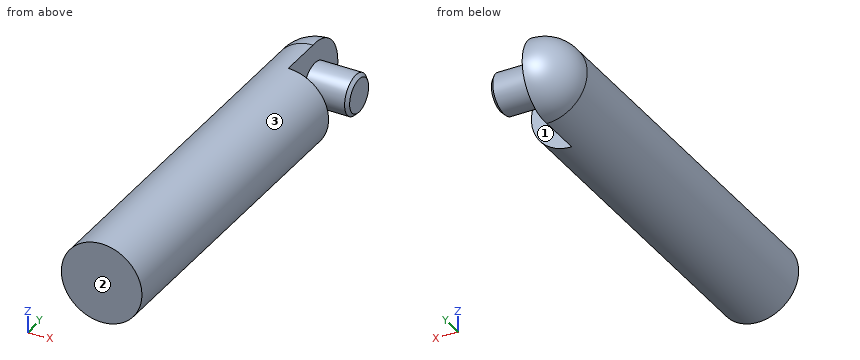
```python
from build123d import *

# Parameters (mm, degrees)
SKETCH1_R               = 19.05
BOSS_EXTRUDE1_DEPTH     = 177.8
DOME1_FACE_RADIUS       = 19.05
DOME1_HEIGHT            = 20.828
CUT_EXTRUDE1_DEPTH      = 201.461172648
CUT_EXTRUDE1_DEPTH_BACK = 201.461172648
SKETCH2_W               = 31.75
SKETCH2_H               = 41.656
SKETCH3_R               = 9.525
BOSS_EXTRUDE2_DEPTH     = 20.828
CHAMFER1_SIZE           = 1.524


with BuildPart() as part:
    # Sketch1 → Boss-Extrude1 (new body)
    with BuildSketch(Plane(origin=(0, 0, 0), x_dir=(1, 0, 0), z_dir=(0, 1, 0))):
        with Locations(Location((0, 0, 0), (0, 0, 270))):
            Circle(SKETCH1_R)
    extrude(amount=BOSS_EXTRUDE1_DEPTH)

    # Dome1: a dome of height H over a round flat face of radius A is a cap of a sphere of radius (A * A + H * H) / (2 * H)
    dome1_r = (DOME1_FACE_RADIUS * DOME1_FACE_RADIUS + DOME1_HEIGHT * DOME1_HEIGHT) / (2 * DOME1_HEIGHT)
    dome1_base = Plane((0, 177.8, 0), z_dir=(0, 1, 0))
    with Locations(dome1_base.offset(DOME1_HEIGHT - dome1_r)):
        dome1_ball = Sphere(dome1_r, mode=Mode.PRIVATE)
    add(split(dome1_ball, bisect_by=dome1_base, keep=Keep.TOP, mode=Mode.PRIVATE))

    # Sketch2 → Cut-Extrude1 (cut, two sides: drawn at the far end of the back side and taken through both)
    with BuildSketch(Plane.XY.offset(-CUT_EXTRUDE1_DEPTH_BACK)):
        with Locations((15.875, 177.8)):
            Rectangle(SKETCH2_W, SKETCH2_H)
    extrude(amount=CUT_EXTRUDE1_DEPTH + CUT_EXTRUDE1_DEPTH_BACK, mode=Mode.SUBTRACT)

    # Sketch3 → Boss-Extrude2 (add)
    with BuildSketch(Plane(origin=(0, 0, 0), x_dir=(0, 0, -1), z_dir=(1, 0, 0))):
        with Locations(Location((0, 179.502109756, 0), (0, 0, 270))):
            Circle(SKETCH3_R)
    extrude(amount=BOSS_EXTRUDE2_DEPTH)

    # Chamfer1
    chamfer1_edges = [part.edges().sort_by_distance(p)[0] for p in [
        (20.828, 189.027109756, 0),
    ]]
    chamfer(chamfer1_edges, length=CHAMFER1_SIZE)


solid = part.part
```
Design review of the part built by this model. Coordinates are the model's own, in mm. Face numbers are marked on the shaded views. Coordinates: 2 decimals unless noted, no trailing zeros. Order: outer loops, then holes, each group sorted by start corner. A loop starts at its lowest first (then second) coordinate and runs counter-clockwise, first axis right, second up.
1) Wall thickness on line 1 along Y through (x, z) = (6.5, -0.5); line 2 along Y through (x, z) = (17, -8.5); line 3 along Z through (x, y) = (-16.5, 135): over which ranges is each line inside the solid? List them lowest first.
2) Take a section at D-D, the plane x = 16.5. Give the boundary of the cut face in (y, z) (3 decimals).
3) Mouldability with a two-part tool opening along Y and no side actions: class the marked faces 1, 2 and 3 as +Y half, -Y half, draft (parallel to the pull), parting line (faces both ways), or undercut.
4) Take a section at C-C, the plane y = 126. Give the boundary of the cut face in (x, z).
5) Take a section at A-A, the plane z = 0. Give the boundary of the cut face in (x, y).
6) Clearance check with flat-ended pins moving along their axes: pin 1 (2 mm diameter, centred on x = -2.5, y = 144.5, fed in from -Z); pin 2 (8 mm diameter, centred on y = 65, z = 5, fed in from -X); pin 3 (3 mm diameter, centred on x = 0, z = 13.5, fed in from -Y); pin 4 (2 mm diameter, centred on x = 5.5, y = 20.5, fed in from +Z). State where each tip first meets the part, or that it passes through.
7) Take a section at B-B, the plane x = 8. Give the boundary of the cut face in (y, z) (3 decimals).
Returned:
1. line 1: y = 0 to 156.97, 169.99 to 189.01
1. line 2: y = 0 to 156.97, 175.2 to 183.8
1. line 3: z = -9.52 to 9.52
2. outline: (0, -9.521) - (156.972, -9.521) - (156.972, 9.521) - (0, 9.521) - close; circle Ø19.05 at (179.502, 0)
3. face 1: undercut
3. face 2: -Y half
3. face 3: draft
4. outline: circle Ø38.1 at (0, 0)
5. outline: (-19.05, 0) - (19.05, 0) - (19.05, 156.97) - (0, 156.97) - (0, 169.98) - (19.3, 169.98) - (20.83, 171.5) - (20.83, 187.5) - (19.3, 189.03) - (0, 189.03) - (0, 198.63) arc R19.13 ccw to (-19.05, 177.8) - close
6. pin 1: stops at z = -18.99
6. pin 2: stops at x = -19.02
6. pin 3: stops at y = 0
6. pin 4: stops at z = 18.51
7. outline: (0, -17.289) - (156.972, -17.289) - (156.972, 17.289) - (0, 17.289) - close; circle Ø19.05 at (179.502, 0)
